from build123d import *

# Parameters (mm, degrees)
F0_W            = 64
F0_H            = 43
F8_DEPTH        = 4
F1_W            = 4
F1_H            = 43
F2_DEPTH        = 43
F4_D            = 4
F9_D            = 23
F5_W            = 39.661507
F5_H            = 43
F10_DEPTH       = 20
F7_D            = 5.5
F7_CBORE_D      = 10
F7_CBORE_DEPTH  = 20
F11_D           = 3.5
F11_CBORE_D     = 5
F11_CBORE_DEPTH = 15
F6_W            = 39.661507
F6_H            = 43
F12_DEPTH       = 15


with BuildPart() as f8:
    # F0 (on Top) → F8 (new body)
    with BuildSketch(Plane.XY):
        Rectangle(F0_W, F0_H)
    extrude(amount=F8_DEPTH)

    # F1 (on face) → F2 (join)
    with BuildSketch(Plane(origin=(0, 0, 0), x_dir=(1, 0, 0), z_dir=(0, 0, -1))):
        with Locations((17, 0)):
            Rectangle(F1_W, F1_H)
    extrude(amount=F2_DEPTH)

    # F4 (through all)
    with Locations(Plane.YZ.offset(19)):
        with Locations((15.5, -37), (15.5, -6), (-15.5, -37), (-15.5, -6)):
            Hole(F4_D / 2)

    # F9 (through all)
    with Locations(Plane.YZ.offset(19)):
        with Locations((0, -21.5)):
            Hole(F9_D / 2)

    # F5 (on face) → F10 (join)
    with BuildSketch(Plane.XY.offset(4)):
        with Locations((-12.169246, 0)):
            Rectangle(F5_W, F5_H)
    extrude(amount=F10_DEPTH)

    # F7 (through all)
    with Locations(Plane.XY.offset(24)):
        with Locations((-18, -15), (-18, 15)):
            CounterBoreHole(F7_D / 2, F7_CBORE_D / 2, F7_CBORE_DEPTH)

    # F11 (through all)
    with Locations(Plane.XY.offset(24)):
        with Locations((-30, 15), (-30, -15)):
            CounterBoreHole(F11_D / 2, F11_CBORE_D / 2, F11_CBORE_DEPTH)

    # F6 (on face) → F12 (cut)
    with BuildSketch(Plane.XY.offset(24)):
        with Locations((-12.169246, 0)):
            Rectangle(F6_W, F6_H)
    extrude(amount=-F12_DEPTH, mode=Mode.SUBTRACT)


solid = f8.part
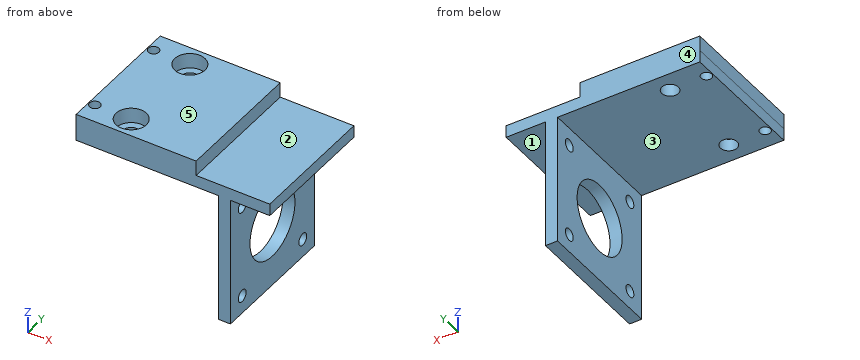
Verification items for the finished model (mm, model axes). Face numbers are marked on the shaded views. A direction names the side the tool comes from. Give positions to 0.01 mm unless a question says otherwise; leave off trailing zeros. Order: outer loops, then holes, each group sorted by start corner. A loop starts at its lowest first (then second) coordinate and runs counter-clockwise, first axis right, second up. Notation, with made-up numbers: (81, 6) -> (133, 6) arc R31 ccw to (133, 42) -> close; hole circle Ø7 at (51, 32.5). An arc over 180 degrees is marked (long way). Answer as CSV lines item,"result".
Q1. Sectioned sample at A-A on y = 0. Record the cut outline in (x, z).
Solutions:
outline,"(-32, 0) -> (15, 0) -> (15, -10) -> (19, -10) -> (19, 0) -> (32, 0) -> (32, 4) -> (7.66, 4) -> (7.66, 9) -> (-32, 9) -> close; (15, -43) -> (19, -43) -> (19, -33) -> (15, -33) -> close"
Q2. Depth check by flat-ended pin: pin 1 (12 mm diameter, centred on x = 17.5, y = -5.5, fed in from +Z); pin 2 (5 mm diameter, centred on y = -5.5, z = -10.5, fed in from -X); pin 3 (6 mm diameter, centred on x = -18, y = 15, fed in from -Z); pin 4 (11 mm diameter, centred on x = -17, y = 17, fed in from +Z). Enter the tip coordinate at first touch or a pass-through.
Solutions:
pin 1,"stops at z = 4"
pin 2,"stops at x = 15"
pin 3,"stops at z = 0"
pin 4,"stops at z = 9"
Q3. Access from +Z, -Z, +X, -X, +Y, -Y to the whole of each face (thin tool, end or side, straight path). Record for the marked faces 1, 2, 3, 4 and 5.
Solutions:
face 1,"-Z, +X, +Y, -Y"
face 2,"+Z, +X, +Y, -Y"
face 3,"-Z, -X, +Y, -Y"
face 4,"+Z, -Z, +X, -X, +Y"
face 5,"+Z, +X, -X, +Y, -Y"
Q4. Sectioned sample at B-B on x = -18. Record the cut outline in (y, z).
Solutions:
outline,"(-21.5, 0) -> (-17.75, 0) -> (-17.75, 4) -> (-20, 4) -> (-20, 9) -> (-21.5, 9) -> close; (-12.25, 0) -> (12.25, 0) -> (12.25, 4) -> (10, 4) -> (10, 9) -> (-10, 9) -> (-10, 4) -> (-12.25, 4) -> close; (17.75, 0) -> (21.5, 0) -> (21.5, 9) -> (20, 9) -> (20, 4) -> (17.75, 4) -> close"
Q5. Sectioned sample at D-D on z = -6. Record the cut outline in (x, y), plus the area to 3 significant figures.
Solutions:
outline,"(15, -21.5) -> (19, -21.5) -> (19, -17.5) -> (15, -17.5) -> close; (15, -13.5) -> (19, -13.5) -> (19, 13.5) -> (15, 13.5) -> close; (15, 17.5) -> (19, 17.5) -> (19, 21.5) -> (15, 21.5) -> close"
area,"140 mm²"
Q6. Sectioned sample at C-C on z = -21.5. Record the cut outline in (x, y), plus the area to 3 significant figures.
Solutions:
outline,"(15, -21.5) -> (19, -21.5) -> (19, -11.5) -> (15, -11.5) -> close; (15, 11.5) -> (19, 11.5) -> (19, 21.5) -> (15, 21.5) -> close"
area,"80.0 mm²"
Q7. Scan lines: probe 1 along Z at (x, y) = (16.5, 15.5); probe 2 along Y at (x, z) = (-30, 6.5); probe 3 along Y at (x, z) = (-19, 3). Record each from-to range of solid material in increasing order.
Solutions:
probe 1,"z = -43 to -39, -35 to -8, -4 to 4"
probe 2,"y = -21.5 to -16.75, -13.25 to 13.25, 16.75 to 21.5"
probe 3,"y = -21.5 to -17.56, -12.44 to 12.44, 17.56 to 21.5"
